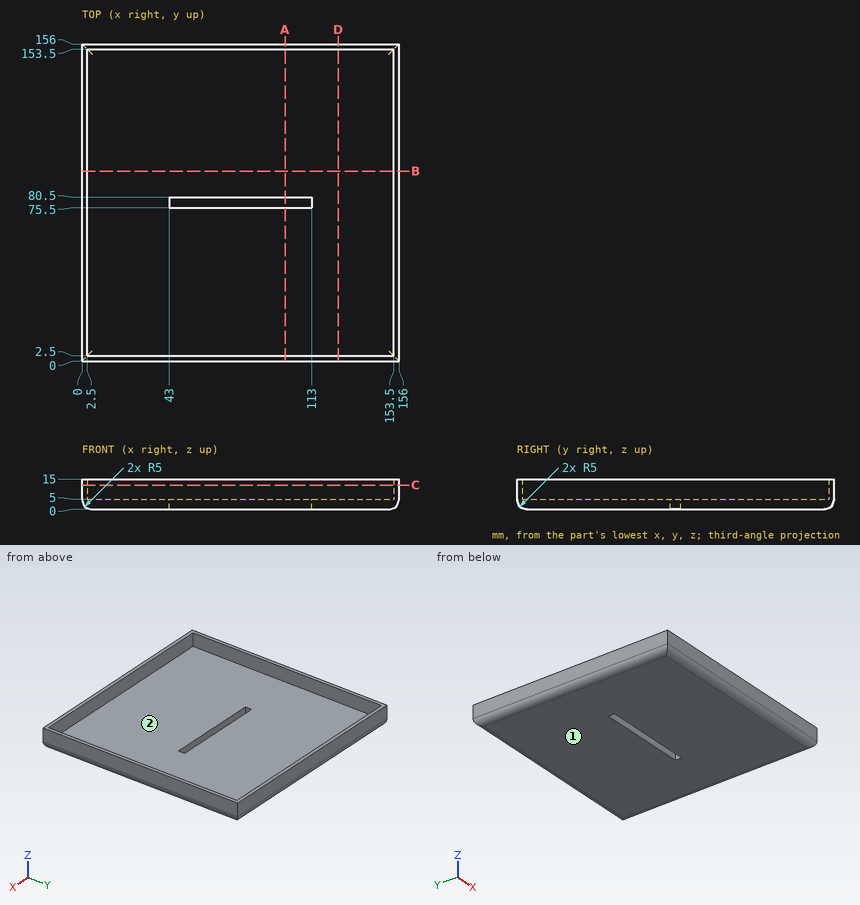
Design review of the part shown in the three views and the two pictorial views. Dimensions are in mm from the part's minimum x, y and z. Coordinates: 2 decimals unless noted, no trailing zeros. Order: outer loops, then holes, each group sorted by start corner. A loop starts at its lowest first (then second) coordinate and runs counter-clockwise, first axis right, second up. Notation, with made-up numbers: (28, -27) - (71, -27) arc R20 ccw to (71, -8) - close; hole circle Ø2 at (13, 26.5). An arc over 180 degrees is marked (long way). Answer as CSV lines item,"result". Start each with the question number.
1) Insertion check: P1, Ø1.5, axis at x = 71, z = 3, coming from the -Y side; P2, Ø1.5, axis at y = 56, z = 7, coming from the -X side; P3, Ø4, axis at y = 77.5, z = 2.5, coming from the +X side; P4, Ø3, axis at y = 127.5, z = 1.5, coming from the +X side. Each pin has a flat end and moves straight along its axis. Give the tip position at first contact, or say it passes through.
2) Add section A-A (x = 100). State the section outline as (y, z) points, then the cut area to 3 significant figures.
3) Add section B-B (y = 93.5). State the section outline as (x, z) points, then the cut area to 3 significant figures.
4) Add section C-C (z = 12). State the section outline as (x, y) points.
5) To check wall thickness, follow line 1 along X through (y, z) = (71, 6.5); line 2 along Z through (x, y) = (58, 136). State the ranges of each line that lie inside material, in increasing order. Write a range as [from, to].
6) Draft analysis for pull direction X (two halves, no side actions). For the marked faces 1 and 2, state which applies: +X half, -X half, draft (parallel to the pull), parting line (faces both ways), or undercut.
Result:
1,P1,"y = 0.16"
1,P2,"x = 0"
1,P3,"x = 155.97"
1,P4,"x = 155.58"
2,outline,"(0, 5) arc R5 ccw to (5, 0) - (75.5, 0) - (75.5, 5) - (2.5, 5) - (2.5, 15) - (0, 15) - close; (80.5, 0) - (151, 0) arc R5 ccw to (156, 5) - (156, 15) - (153.5, 15) - (153.5, 5) - (80.5, 5) - close"
2,area,"794 mm^2"
3,outline,"(0, 5) arc R5 ccw to (5, 0) - (151, 0) arc R5 ccw to (156, 5) - (156, 15) - (153.5, 15) - (153.5, 5) - (2.5, 5) - (2.5, 15) - (0, 15) - close"
3,area,"819 mm^2"
4,outline,"(0, 0) - (156, 0) - (156, 156) - (0, 156) - close; hole (2.5, 2.5) - (153.5, 2.5) - (153.5, 153.5) - (2.5, 153.5) - close"
5,line 1,"[0, 2.5], [153.5, 156]"
5,line 2,"[0, 5]"
6,face 1,"draft"
6,face 2,"undercut"
